from build123d import *

# Parameters (mm, degrees)
BOSS_EXTRUDE1_DEPTH = 18
SKETCH2_R           = 1.5
SKETCH2_W           = 30
SKETCH2_H           = 2.78
CUT_EXTRUDE1_DEPTH  = 6.57
SKETCH3_W           = 3.1
SKETCH3_H           = 6.15
CUT_EXTRUDE2_DEPTH  = 6.57
SKETCH4_W           = 3
SKETCH4_H           = 7.645
CUT_EXTRUDE3_DEPTH  = 4.57


with BuildPart() as part:
    # Sketch1 → Boss-Extrude1 (new body, symmetric)
    with BuildSketch(Plane(origin=(0, 0, 0), x_dir=(0, 0, -1), z_dir=(1, 0, 0))):
        Polygon((0, 0), (0, 40.35), (-2, 40.35), (-2, 9.45), (-5.57, 2.78), (-2, 2.78), (-2, 0), align=None)
    extrude(amount=BOSS_EXTRUDE1_DEPTH, both=True)

    # Sketch2 → Cut-Extrude1 (cut, through all)
    with BuildSketch(Plane(origin=(0, 0, 0), x_dir=(-1, 0, 0), z_dir=(0, 0, -1))):
        with Locations((0, 37.1)):
            Circle(SKETCH2_R)
        with Locations((0, 1.39)):
            Rectangle(SKETCH2_W, SKETCH2_H)
    extrude(amount=-CUT_EXTRUDE1_DEPTH, mode=Mode.SUBTRACT)

    # Sketch3 → Cut-Extrude2 (cut, through all)
    with BuildSketch(Plane(origin=(0, 0, 0), x_dir=(-1, 0, 0), z_dir=(0, 0, -1))):
        with Locations((-16.45, 13.5)):
            Rectangle(SKETCH3_W, SKETCH3_H)
        with Locations((16.45, 13.5)):
            Rectangle(SKETCH3_W, SKETCH3_H)
    extrude(amount=-CUT_EXTRUDE2_DEPTH, mode=Mode.SUBTRACT)

    # Sketch4 → Cut-Extrude3 (cut, through all)
    with BuildSketch(Plane.XY.offset(2)):
        with Locations((-16.5, 6.6025)):
            Rectangle(SKETCH4_W, SKETCH4_H)
        with Locations((16.5, 6.6025)):
            Rectangle(SKETCH4_W, SKETCH4_H)
    extrude(amount=CUT_EXTRUDE3_DEPTH, mode=Mode.SUBTRACT)


solid = part.part
Source: CAD feature listing. Evaluate the final solid. Frame: model axes, mm. A direction names the side the tool comes from. Round coordinates to 2 decimals unless told otherwise and drop trailing zeros. Write each loop counter-clockwise with the first axis right and the second up, starting at its lowest first coordinate (ties: lowest second). Pieces come first, ordered by that corner, then holes. Notation, with made-up numbers: (-24, 60.5) - (-13, 60.5) arc R21 cw to (-13, 70.5) - close; hole circle Ø6 at (28, 57.25). An arc over 180 degrees is marked (long way). Use CSV: the item, a comma, the result in double quotes. Start each with the question number.
(1) Cut plane B-B, the plane x = 0. Return loops of the section in (y, z), and give its area (3 significant figures).
(2) Cut plane D-D, the plane y = 28. Return loops of the section in (x, z).
(3) Material intervals for probe 1 along Y at (x, z) = (0, 0.7); probe 2 along Z at (x, y) = (4, 31); probe 3 along Y at (x, z) = (2, 0.9), sorted ascending. Write a range as [from, to].
(4) Cut plane A-A, the plane y = 37.1. Return loops of the section in (x, z), and give its area (3 significant figures).
(5) First-contact query: pin 1 Ø1.8 at (y, z) = (6, 3) entering from +X; pin 2 Ø1.1 at (y, z) = (7.5, 4) entering from -X; pin 3 Ø1.6 at (y, z) = (13, 0.5) entering from -X; pin 4 Ø1 at (y, z) = (14.5, 1) entering from +X. Flat tips, straight axial feed; report the tip coordinate or a pass-through.
(6) Mould query, pull axis X, two halves, no side actions, for faces 4 (the face through (-15, 1, 1)), 5 (the face through (-15, 5, 3)), 6 (the face through (0, 2.78, 3)), 7 (the face through (-16, 10.425, 1)). Classes: pulls with the +X half, pulls with the -X half, needs draft (parallel to the pull), parting line crosses it, or undercut.
(7) Cut plane C-C, the plane x = -9. Return loops of the section in (y, z), and give its area (3 significant figures).
(8) Set-up query: faces 1 (the face through (-14.9, 13, 1)), 2 (the face through (0.21, 6.16, 3.76)), 3 (the face through (16, 16.575, 1)). Return all of +Z, -Z, +X, -X, +Y, -Y with unobstructed straight access to the full face (end or side cutting, diameter ignored); none if empty.
Geometry says:
1,outline,"(2.78, 0) - (35.6, 0) - (35.6, 2) - (9.45, 2) - (2.78, 5.57) - close; (38.6, 0) - (40.35, 0) - (40.35, 2) - (38.6, 2) - close"
1,area,"81.0 mm²"
2,outline,"(-18, 0) - (18, 0) - (18, 2) - (-18, 2) - close"
3,probe 1,"[2.78, 35.6], [38.6, 40.35]"
3,probe 2,"[0, 2]"
3,probe 3,"[2.78, 40.35]"
4,outline,"(-18, 0) - (-1.5, 0) - (-1.5, 2) - (-18, 2) - close; (1.5, 0) - (18, 0) - (18, 2) - (1.5, 2) - close"
4,area,"66.0 mm²"
5,pin 1,"x = 15"
5,pin 2,"through"
5,pin 3,"x = -14.9"
5,pin 4,"x = 14.9"
6,face 4,"undercut"
6,face 5,"pulls with the -X half"
6,face 6,"undercut"
6,face 7,"needs draft"
7,outline,"(2.78, 0) - (40.35, 0) - (40.35, 2) - (9.45, 2) - (2.78, 5.57) - close"
7,area,"87.0 mm²"
8,face 1,"+Z, -Z, -X"
8,face 2,"+Z, +X, -X, +Y"
8,face 3,"+Z, -Z, +X"
